```python
from build123d import *

# Parameters (mm, degrees)
SKETCH1_R           = 2.1
BOSS_EXTRUDE1_DEPTH = 1.5


with BuildPart() as part:
    # Sketch1 → Boss-Extrude1 (new body)
    with BuildSketch(Plane.XY):
        with BuildLine():
            Line((-17.5, -5), (17.5, -5))
            ThreePointArc((17.5, -5), (18.207106781, -4.707106781), (18.5, -4))
            Line((18.5, -4), (18.5, 4))
            ThreePointArc((18.5, 4), (18.207106781, 4.707106781), (17.5, 5))
            Line((17.5, 5), (-17.5, 5))
            ThreePointArc((-17.5, 5), (-18.207106781, 4.707106781), (-18.5, 4))
            Line((-18.5, 4), (-18.5, -4))
            ThreePointArc((-18.5, -4), (-18.207106781, -4.707106781), (-17.5, -5))
        make_face()
        with Locations(Location((-10, 0, 0), (0, 0, 180))):
            Circle(SKETCH1_R, mode=Mode.SUBTRACT)
        with Locations(Location((10, 0, 0), (0, 0, 180))):
            Circle(SKETCH1_R, mode=Mode.SUBTRACT)
    extrude(amount=BOSS_EXTRUDE1_DEPTH)


solid = part.part
```
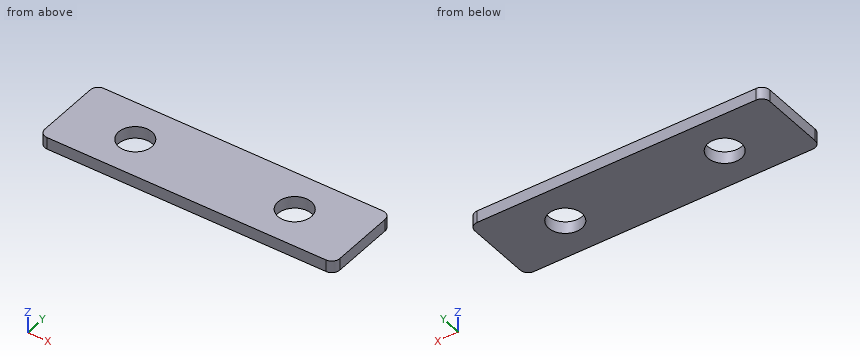
Design review of the part built by this model. Coordinates are the model's own, in mm. Give positions to 0.01 mm unless a question says otherwise; leave off trailing zeros. Write each loop counter-clockwise with the first axis right and the second up, starting at its lowest first coordinate (ties: lowest second). Pieces come first, ordered by that corner, then holes. Notation, with made-up numbers: (21, -25) -> (45, -25) arc R11 cw to (45, -6) -> close; hole circle Ø4 at (68, 19.5). An arc over 180 degrees is marked (long way). Answer in a Markdown table with one row per item.
(1) To check wall thickness, follow probe 1 along Y at (x, z) = (-10, 0.9); probe 2 along X at (y, z) = (1, 0.85); probe 3 along Y at (x, z) = (-9.5, 0.9). State the ranges of each line that lie inside material, in increasing order.
Results:
| item | result |
|---|---|
| probe 1 | -5 to -2.1, 2.1 to 5 |
| probe 2 | -18.5 to -11.85, -8.15 to 8.15, 11.85 to 18.5 |
| probe 3 | -5 to -2.04, 2.04 to 5 |
(2) Consider section C-C (z = 0.9). State the section outline as (x, y) points.
Results:
| item | result |
|---|---|
| outline | (-18.5, -4) arc R1 ccw to (-17.5, -5) -> (17.5, -5) arc R1 ccw to (18.5, -4) -> (18.5, 4) arc R1 ccw to (17.5, 5) -> (-17.5, 5) arc R1 ccw to (-18.5, 4) -> close; hole circle Ø4.2 at (-10, 0); hole circle Ø4.2 at (10, 0) |
(3) Clearance check with a flat-ended pin moving along its axis: pin 1 (5 mm diameter, centred on x = 7.5, y = 1.5, fed in from -Z). State where the tip first meets the part, or that it passes through.
Results:
| item | result |
|---|---|
| pin 1 | z = 0 |
(4) Consider section D-D (x = 9). State the section outline as (y, z) points.
Results:
| item | result |
|---|---|
| outline | (-5, 0) -> (-1.85, 0) -> (-1.85, 1.5) -> (-5, 1.5) -> close; (1.85, 0) -> (5, 0) -> (5, 1.5) -> (1.85, 1.5) -> close |
(5) Consider section B-B (x = -10). State the section outline as (y, z) points.
Results:
| item | result |
|---|---|
| outline | (-5, 0) -> (-2.1, 0) -> (-2.1, 1.5) -> (-5, 1.5) -> close; (2.1, 0) -> (5, 0) -> (5, 1.5) -> (2.1, 1.5) -> close |
(6) Consider section A-A (y = 0). State the section outline as (x, z) points, then the cut area to 3 significant figures.
Results:
| item | result |
|---|---|
| outline | (-18.5, 0) -> (-12.1, 0) -> (-12.1, 1.5) -> (-18.5, 1.5) -> close; (-7.9, 0) -> (7.9, 0) -> (7.9, 1.5) -> (-7.9, 1.5) -> close; (12.1, 0) -> (18.5, 0) -> (18.5, 1.5) -> (12.1, 1.5) -> close |
| area | 42.9 mm2 |
